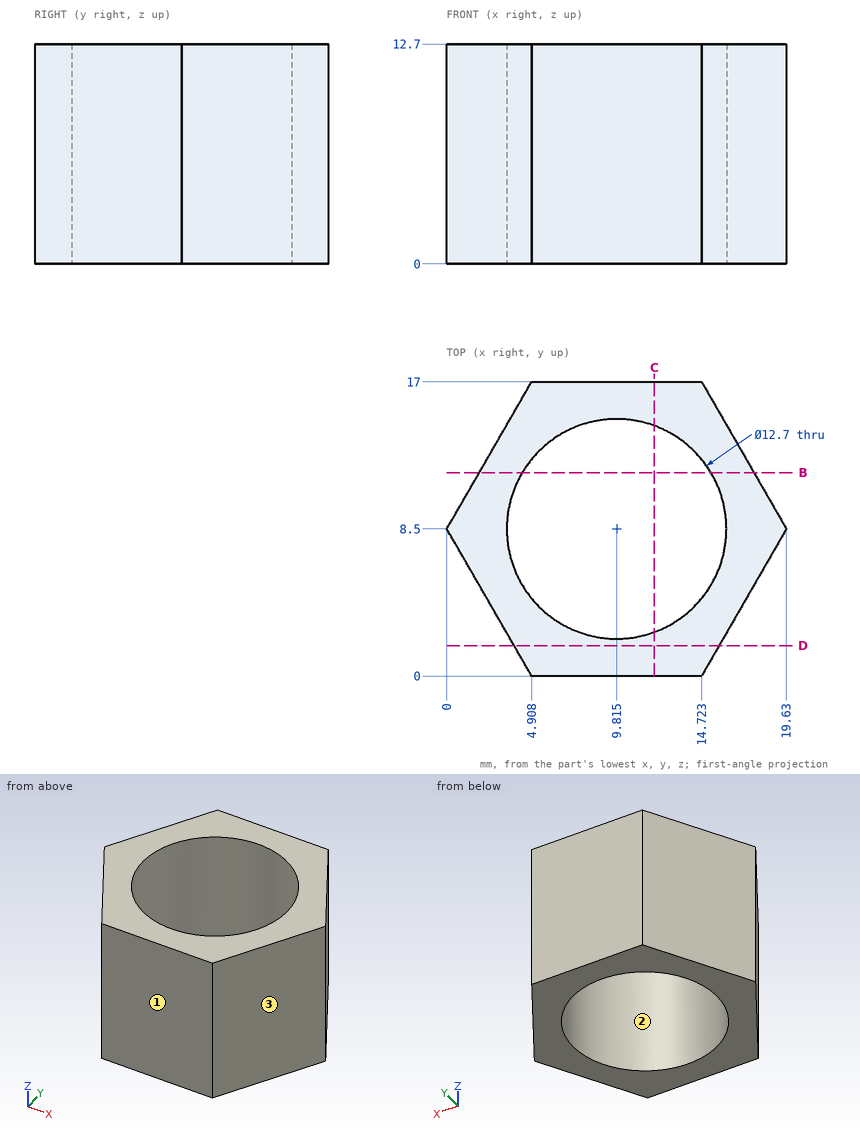
Here's the drawing with two shaded views (mm, measured from the low corner). I have some questions. Coordinates: 2 decimals unless noted, no trailing zeros. Order: outer loops, then holes, each group sorted by start corner. A loop starts at its lowest first (then second) coordinate and runs counter-clockwise, first axis right, second up. Notation, with made-up numbers: (68.25, 44) - (109.25, 44) arc R11 ccw to (109.25, 60) - close; hole circle Ø11 at (-28.75, 65.25). An arc over 180 degrees is marked (long way). Answer in a Markdown table with one row per item. Add a question column.
(1) If we mould it in two halves opening along X, with no side actions, what happens to the marked faces 1, 2 and 3? For each: released by +X, released by -X, zero draft, split by the parting line, or undercut.
(2) I need wall thicknesses on L1, parallel to Y at x = 10, z = 7.25; L2, parallel to Y at x = 7.25, z = 0.5; L3, parallel to X at y = 13.5, z = 7.5 (1 decimal). Which ranges of each line are inside material? Lowest first, please.
(3) If we section it at B-B, the plane y = 11.75: Please give me the cut outline in (x, z).
(4) If we section it at C-C, the plane x = 12: Please give me the cut outline in (y, z).
(5) Will these pins go through, and if not, where does the flat tip stop? pin 1 (6 mm diameter, centred on y = 12.5, z = 5, fed in from -X); pin 2 (1 mm diameter, centred on y = 4.5, z = 5, fed in from +X); pin 3 (3 mm diameter, centred on y = 11.5, z = 11.5, fed in from -X) (1 decimal).
(6) If we section it at D-D, the plane y = 1.75: Please give me the cut outline in (x, z).
Results are:
| question | item | result |
|---|---|---|
| 1 | face 1 | zero draft |
| 1 | face 2 | undercut |
| 1 | face 3 | released by +X |
| 2 | L1 | y = 0 to 2.15, 14.85 to 17 |
| 2 | L2 | y = 0 to 2.69, 14.31 to 17 |
| 2 | L3 | x = 2.9 to 5.9, 13.7 to 16.7 |
| 3 | outline | (1.88, 0) - (4.36, 0) - (4.36, 12.7) - (1.88, 12.7) - close; (15.27, 0) - (17.75, 0) - (17.75, 12.7) - (15.27, 12.7) - close |
| 4 | outline | (0, 0) - (2.54, 0) - (2.54, 12.7) - (0, 12.7) - close; (14.46, 0) - (17, 0) - (17, 12.7) - (14.46, 12.7) - close |
| 5 | pin 1 | stops at x = 0.58 |
| 5 | pin 2 | stops at x = 17.61 |
| 5 | pin 3 | stops at x = 0.9 |
| 6 | outline | (3.9, 0) - (15.73, 0) - (15.73, 12.7) - (3.9, 12.7) - close |
